Design review of the part built by this model. Coordinates are the model's own, in mm. Give positions to 0.01 mm unless a question says otherwise; leave off trailing zeros. Write each loop counter-clockwise with the first axis right and the second up, starting at its lowest first coordinate (ties: lowest second). Pieces come first, ordered by that corner, then holes. Notation, with made-up numbers: (-33, -11) - (16, -11) arc R24 ccw to (16, 8) - close; hole circle Ø4 at (75, -28.75). An arc over 180 degrees is marked (long way). Write each question's results on one line, items separated by ' | '. Start each with the question number.
from build123d import *

# Parameters (mm, degrees)
F1_DEPTH = 3.302


with BuildPart() as f1:
    # F0 (on Top) → F1 (new body)
    with BuildSketch(Plane.XY):
        Polygon((-7.29726, 50.8), (-38.1, 50.8), (-38.1, 57.15), (-50.8, 57.15), (-50.8, 50.8), (-57.15, 50.8), (-57.15, 38.1), (-50.8, 38.1), (-50.8, 6.698998), (-57.15, 6.698998), (-57.15, -6.001002), (-50.8, -6.001002), (-50.8, -38.1), (-57.15, -38.1), (-57.15, -50.8), (-50.8, -50.8), (-50.8, -57.15), (-38.1, -57.15), (-38.1, -50.8), (-7.29726, -50.8), (-7.29726, -57.15), (5.40274, -57.15), (5.40274, -50.8), (38.1, -50.8), (38.1, -57.15), (50.8, -57.15), (50.8, -50.8), (57.15, -50.8), (57.15, -38.1), (50.8, -38.1), (50.8, -6.001002), (57.15, -6.001002), (57.15, 6.698998), (50.8, 6.698998), (50.8, 38.1), (57.15, 38.1), (57.15, 50.8), (50.8, 50.8), (50.8, 57.15), (38.1, 57.15), (38.1, 50.8), (5.40274, 50.8), (5.40274, 57.15), (-7.29726, 57.15), align=None)
    extrude(amount=F1_DEPTH)


solid = f1.part
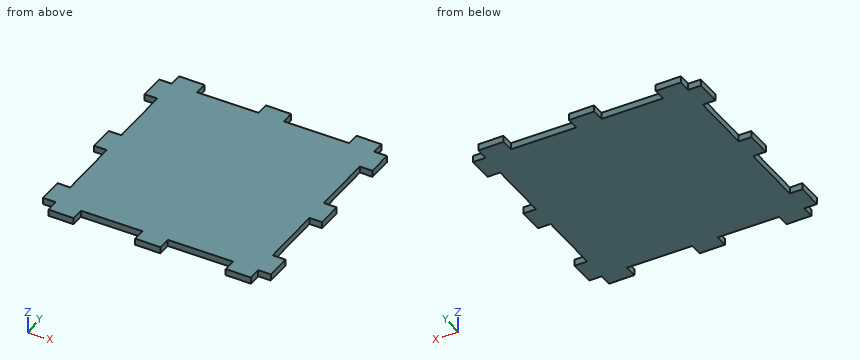
Q1. Insertion check: P1, Ø1, axis at x = -20, z = 1, coming from the -Y side; P2, Ø1, axis at y = 19, z = 2.5, coming from the -X side; P3, Ø1, axis at x = -53.5, z = 1, coming from the +Y side. Each pin has a flat end and moves straight along its axis. Give the tip position at first contact, or say it passes through.
Q2. Add section A-A on y = -34.5. State the section outline as (x, z) points.
Q3. For line 1 along Y through (x, z) = (-51.5, 0.85); line 2 along X through (y, z) = (22, 1.6), list the stretches that pass through material, from the lowest coordinate up. Write a range as [from, to].
Result:
1) P1: stops at y = -50.8 | P2: stops at x = -50.8 | P3: stops at y = 50.8
2) outline: (-50.8, 0) - (50.8, 0) - (50.8, 3.3) - (-50.8, 3.3) - close
3) line 1: y = [-50.8, -38.1], [-6, 6.7], [38.1, 50.8] | line 2: x = [-50.8, 50.8]
